The listing builds one solid part. Answer for the finished solid, in the listing's coordinates (mm). A direction names the side the tool comes from. Round coordinates to 2 decimals unless told otherwise and drop trailing zeros. Write each loop counter-clockwise with the first axis right and the second up, starting at its lowest first coordinate (ties: lowest second). Pieces come first, ordered by that corner, then holes. Notation, with made-up numbers: (5, -11.75) - (53, -11.75) arc R25 cw to (53, 11.25) - close; hole circle Ø3 at (-8, 26). An arc over 180 degrees is marked (long way). Return JSON: item names as keys, results as strings. Group by question number.
(1) Section D-D, the plane y = 0 is taken. Write down the section's boundary in (x, z), then the cut area to 3 significant figures.
(2) Find the intervals of material crossed by line 1 along Y through (x, z) = (2.5, 10.75); line 2 along X through (y, z) = (-1.75, 2.5); line 3 along X through (y, z) = (-2, 3.75), in increasing order. Write a range as [from, to].
(3) Each of these flat-tipped pins is pushed along its axis until it touches: pin 1 (3 mm diameter, centred on y = -3, z = 4.5, fed in from -X); pin 2 (1.8 mm diameter, centred on y = 4, z = 6, fed in from -X); pin 3 (1 mm diameter, centred on y = 2.5, z = 12.5, fed in from -X). Where does it stop, or does it pass through?
(4) Section A-A, the plane x = 2.5 is taken. Write down the section's boundary in (y, z), then the cut area to 3 significant figures.
(5) Which of the six approach directions +Z, -Z, +X, -X, +Y, -Y give full straight-line access (tool end or side, diameter ignored) to faces 5 (the cylindrical face through (-3.058, -4.507, 4.078)), 6 (the cylindrical face through (7.6, 3, 7.4)), 7 (the flat face through (-5, 0, 0))?
(6) Section C-C, the plane x = -3.5 is taken. Write down the section's boundary in (y, z), then the cut area to 3 significant figures.
(7) Determine the mould class of faces 1 (the flat face through (0, 5, 7)), 2 (the flat face through (10, 4, 7)), 3 (the cylindrical face through (-12.46, 2.85, 7.4)), 4 (the cylindrical face through (-0.5, -0.1, 7.4)) for opening direction X: +X half, -X half, draft (parallel to the pull), parting line (faces both ways), or undercut.
```python
from build123d import *

# Parameters (mm, degrees)
F1_DEPTH = 15
F2_R     = 1.5
F3_DEPTH = 1


with BuildPart() as f1:
    # F0 (on Top) → F1 (new body)
    with BuildSketch(Plane.XY):
        with BuildLine():
            Line((-10, -5), (10, -5))
            Line((10, -5), (10, -2.459675))
            ThreePointArc((10, -2.459675), (9.822474, -2.185813), (9.5, -2.236068))
            ThreePointArc((9.5, -2.236068), (7.581884, -2.998882), (5.625, -2.341874))
            ThreePointArc((5.625, -2.341874), (5, -2.122499), (4.375, -2.341874))
            ThreePointArc((4.375, -2.341874), (-0.5, 0), (4.375, 2.341874))
            ThreePointArc((4.375, 2.341874), (5, 2.122499), (5.625, 2.341874))
            ThreePointArc((5.625, 2.341874), (7.581884, 2.998882), (9.5, 2.236068))
            ThreePointArc((9.5, 2.236068), (9.822474, 2.185813), (10, 2.459675))
            Line((10, 2.459675), (10, 5))
            Line((10, 5), (-10, 5))
            Line((-10, 5), (-10, 1.368393))
            ThreePointArc((-10, 1.368393), (-12.5, 2.85), (-15, 1.368393))
            ThreePointArc((-15, 1.368393), (-20.35, 0), (-15, -1.368393))
            ThreePointArc((-15, -1.368393), (-12.5, -2.85), (-10, -1.368393))
            Line((-10, -1.368393), (-10, -5))
        make_face()
    extrude(amount=F1_DEPTH)

    # F2 (on face) → F3 (cut)
    with BuildSketch(Plane.XZ.offset(5)):
        with Locations((-4.443438, 4.652022)):
            Circle(F2_R)
    extrude(amount=-F3_DEPTH, mode=Mode.SUBTRACT)


solid = f1.part
```
Working result:
{
 "1": {"outline": "(-20.35, 0) - (-0.5, 0) - (-0.5, 15) - (-20.35, 15) - close", "area": "298 mm^2"},
 "2": {"line 1": "y = [-5, -3], [3, 5]", "line 2": "x = [-19.75, -15.25], [-14.75, -10.25], [-10, 0.06]", "line 3": "x = [-19.53, -15.47], [-14.53, -10.47], [-10, 0.26]"},
 "3": {"pin 1": "stops at x = -19.92", "pin 2": "stops at x = -10", "pin 3": "stops at x = -19.53"},
 "4": {"outline": "(-5, 0) - (-3, 0) - (-3, 15) - (-5, 15) - close; (3, 0) - (5, 0) - (5, 15) - (3, 15) - close", "area": "60.0 mm^2"},
 "5": {"face 5": "-Y", "face 6": "+Z, -Z", "face 7": "-Z, +X, -X, +Y, -Y"},
 "6": {"outline": "(-5, 0) - (5, 0) - (5, 15) - (-5, 15) - (-5, 5.82) - (-4, 5.82) - (-4, 3.49) - (-5, 3.49) - close", "area": "148 mm^2"},
 "7": {"face 1": "draft", "face 2": "+X half", "face 3": "undercut", "face 4": "undercut"}
}
